CAD build for the part. Positions are in the model's coordinates, mm. A direction names the side the tool comes from. Coordinates: 2 decimals unless noted, no trailing zeros. Write each loop counter-clockwise with the first axis right and the second up, starting at its lowest first coordinate (ties: lowest second). Pieces come first, ordered by that corner, then holes. Notation, with made-up numbers: M 57,75.25 L 77,75.25 A22 cw 77,94.25 Z; hole C -36,23 d11. An arc over 180 degrees is marked long. Answer as CSV lines item,"result". Start each with the question number.
```python
from build123d import *

# Parameters (mm, degrees)
F1_DEPTH  = 22.225
F3_DEPTH  = 1.905
F5_DEPTH  = 38.1
F7_ANGLE  = 90
F9_DEPTH  = 31.75
F11_START = 27.5250845814
F10_R     = 25.4
F11_DEPTH = 40.1837304781


with BuildPart() as f1:
    # F0 (on Right) → F1 (new body, symmetric)
    with BuildSketch(Plane.YZ):
        with BuildLine():
            ThreePointArc((2.9197783942, -1.2472045256), (3.1105402587, -0.6365251756), (3.175, 0))
            ThreePointArc((3.175, 0), (-2.1065171016, 2.3755442957), (-0.3797783942, -3.1522045256))
            ThreePointArc((-0.3797783942, -3.1522045256), (1.5875, -2.749630657), (2.9197783942, -1.2472045256))
        make_face()
        with BuildLine():
            ThreePointArc((2.9197783942, -1.2472045256), (1.5875, -2.749630657), (-0.3797783942, -3.1522045256))
            Line((-0.3797783942, -3.1522045256), (25.0202216058, -47.1462950379))
            Line((25.0202216058, -47.1462950379), (28.3197783942, -45.2412950379))
            Line((28.3197783942, -45.2412950379), (2.9197783942, -1.2472045256))
        make_face()
    extrude(amount=F1_DEPTH, both=True)

    # F2 (on Right) → F3 (join, symmetric)
    with BuildSketch(Plane.YZ):
        with BuildLine():
            Line((26.4980818491, -46.2930520286), (4.9071120764, -8.8963953976))
            ThreePointArc((4.9071120764, -8.8963953976), (2.5335965307, -9.8390288453), (0, -10.16))
            Line((0, -10.16), (-12.7, -10.16))
            Line((-12.7, -10.16), (-12.7, -53.3403694007))
            Line((-12.7, -53.3403694007), (0, -53.3403694007))
            ThreePointArc((0, -53.3403694007), (13.7096045149, -51.5484408285), (26.4980818491, -46.2930520286))
        make_face()
    extrude(amount=F3_DEPTH, both=True)

    # F4 (on Right) → F5 (intersect, symmetric)
    with BuildSketch(Plane.YZ):
        with BuildLine():
            Line((-12.7, -22.225), (0, -22.225))
            ThreePointArc((0, -22.225), (21.2050948807, 6.6554170492), (-12.7, 18.2389864028))
            Line((-12.7, 18.2389864028), (-12.7, -22.225))
        make_face()
    extrude(amount=F5_DEPTH, both=True, mode=Mode.INTERSECT)

    # F6 (on Front) → F7 (revolve, cut)
    with BuildSketch(Plane.XZ):
        with BuildLine():
            Line((29.537089169, 0), (22.098, 0))
            ThreePointArc((22.098, 0), (0, -22.098), (-22.098, 0))
            Line((-22.098, 0), (-30.2814375609, 0))
            Line((-30.2814375609, 0), (-30.2814375609, -27.1878223866))
            Line((-30.2814375609, -27.1878223866), (29.537089169, -27.1878223866))
            Line((29.537089169, -27.1878223866), (29.537089169, 0))
        make_face()
    revolve(axis=Axis((11.049, 0, 0), (1, 0, 0)), revolution_arc=F7_ANGLE, mode=Mode.SUBTRACT)

    # F8 (on Right) → F9 (join, symmetric)
    with BuildSketch(Plane.YZ):
        Polygon((-23.5796823341, 25.4), (-27.5240845814, 25.4), (-14.7630042919, -22.225), (-12.7, -22.225), (-12.7, -7.62), (-14.732, -7.62), align=None)
        Polygon((-12.7, -22.225), (-14.7630042919, -22.225), (-13.9122656059, -25.4), (-11.9874563975, -24.884248927), align=None)
    extrude(amount=F9_DEPTH, both=True)

    # F10 (on Front) → F11 (intersect)
    with BuildSketch(Plane.XZ.offset(F11_START)):
        Circle(F10_R)
    extrude(amount=-F11_DEPTH, mode=Mode.INTERSECT)


solid = f1.part
```
1) Band-saw the part on C-C, the plane y = 2. List the corners of the cut face in (x, z) (3 decimals), plus the area to 3 significant figures.
2) Tool access for faces 5 (the flat face through (0.36, -18.11, 4.99)), 6 (the flat face through (0, -12.7, -10)), 7 (the flat face through (22.225, -1, 1)), 8 (the flat face through (0.07, -12.75, -25.09)), 9 (the cylindrical face through (0.3, -1.5, 2.8)): list every direction of +Z, -Z, +X, -X, +Y, -Y with a clear straight run to the whole face (end or side of a thin tool).
3) Two-plate mould, pull along Y, no slides. Class faces 1 (the flat face through (0, -6, -10.16)), 2 (the flat face through (0.306, 6.775, -7.924)), 3 (the flat face through (-22.225, -1, 1)), 4 (the flat face through (0, -14, -7.62)): pulls with the +Y half, pulls with the -Y half, needs draft (parallel to the pull), parting line crosses it, or undercut.
4) Band-saw the part on D-D, the plane x = 6. List the corners of the cut face in (y, z) (3 decimals), plus the area to 3 significant figures.
5) Pin check, flat tips, straight feed: P1, Ø10, axis at x = 1, z = 19.5, coming from the +Y side; P2, Ø3, axis at x = -0.5, y = -3.5, coming from the +Z side; P3, Ø1.5, axis at x = 6.5, y = 1.5, coming from the -Z side. Stop position of each tip, or through.
6) Probe L1, parallel to Y at x = 9.5, z = 1; L2, parallel to Y at x = 8.5, z = -11; L3, parallel to X at y = -8.5, z = -16 (3 decimals). List the from-to ranges inside material, lowest first. Write a range as [from, to].
7) Band-saw the part on B-B, the plane z = -6.5. List the corners of the cut face in (x, y), plus the area to 3 significant figures.
Result sheet:
1,outline,"M -22.225,0 L -22.007,0 A22.007 ccw -20.77,-7.274 L 20.77,-7.274 A22.007 ccw 22.007,0 L 22.225,0 L 22.225,2.466 L -22.225,2.466 Z; M -1.905,-21.925 A22.007 ccw 1.905,-21.925 L 1.905,-9.961 L -1.905,-9.961 Z"
1,area,"470 mm²"
2,face 5,"+Z, +X, -X"
2,face 6,"+Z"
2,face 7,"+Z, -Z, +X, +Y"
2,face 8,"-Z, +X, -X, +Y"
2,face 9,"+X, -X"
3,face 1,"undercut"
3,face 2,"pulls with the +Y half"
3,face 3,"needs draft"
3,face 4,"undercut"
4,outline,"M -27.331,24.681 L -14.105,-24.681 L -12.042,-24.681 L -12.7,-22.225 L -12.7,-7.62 L -14.732,-7.62 L -23.387,24.681 Z; M -0.38,-3.152 L 8.941,-19.297 A21.268 ccw 12.241,-17.392 L 2.92,-1.247 A3.175 ccw long Z"
4,area,"292 mm²"
5,P1,"stops at y = -20.66"
5,P2,"stops at z = 2.47"
5,P3,"stops at z = -7.71"
6,L1,"y = [-20.99, -17.04], [-3.01, 3.01]"
6,L2,"y = [-17.77, -12.7], [4.15, 8.55]"
6,L3,"x = [-1.905, 1.905]"
7,outline,"M -24.55,-18.98 L 24.55,-18.98 L 24.55,-15.03 L -24.55,-15.03 Z; M -21.06,1.55 L 21.06,1.55 A21.12 ccw 20.26,5.95 L -20.26,5.95 A21.12 ccw Z"
7,area,"376 mm²"
